```python
from build123d import *

# Parameters (mm, degrees)
SKETCH1_W                   = 231.775
SKETCH1_H                   = 298.45
BOSS_EXTRUDE1_DEPTH         = 3.175
F_1_4_0_25_DIAMETER_HOLE1_D = 6.35
FILLET1_R                   = 3.175
SKETCH4_W                   = 12.7
SKETCH4_H                   = 19.05
CUT_EXTRUDE1_DEPTH          = 4.175
FILLET2_R                   = 1.905


with BuildPart() as part:
    # Sketch1 → Boss-Extrude1 (new body)
    with BuildSketch(Plane(origin=(0, 0, 0), x_dir=(1, 0, 0), z_dir=(0, 1, 0))):
        Rectangle(SKETCH1_W, SKETCH1_H)
    extrude(amount=BOSS_EXTRUDE1_DEPTH)

    # 1/4 (0.25) Diameter Hole1 (through all)
    with Locations(Plane(origin=(0, 3.175, 0), x_dir=(1, 0, 0), z_dir=(0, 1, 0))):
        with Locations((61.9125, 0)):
            Hole(F_1_4_0_25_DIAMETER_HOLE1_D / 2)

    # Fillet1
    fillet1_edges = [part.edges().sort_by_distance(p)[0] for p in [
        (115.8875, 1.5875, 149.225),
        (-115.8875, 1.5875, 149.225),
        (-115.8875, 1.5875, -149.225),
        (115.8875, 1.5875, -149.225),
    ]]
    fillet(fillet1_edges, radius=FILLET1_R)

    # Sketch4 → Cut-Extrude1 (cut, through all)
    with BuildSketch(Plane(origin=(0, 3.175, 0), x_dir=(1, 0, 0), z_dir=(0, 1, 0))):
        with Locations((61.9125, -114.3)):
            Rectangle(SKETCH4_W, SKETCH4_H)
        with Locations((61.9125, 114.3)):
            Rectangle(SKETCH4_W, SKETCH4_H)
    extrude(amount=-CUT_EXTRUDE1_DEPTH, mode=Mode.SUBTRACT)

    # Fillet2
    fillet2_edges = [part.edges().sort_by_distance(p)[0] for p in [
        (55.5625, 1.5875, 123.825),
        (55.5625, 1.5875, 104.775),
        (68.2625, 1.5875, 104.775),
        (68.2625, 1.5875, 123.825),
        (55.5625, 1.5875, -104.775),
        (55.5625, 1.5875, -123.825),
        (68.2625, 1.5875, -123.825),
        (68.2625, 1.5875, -104.775),
    ]]
    fillet(fillet2_edges, radius=FILLET2_R)


solid = part.part
```
CAD build for the part. Positions are in the model's coordinates, mm. Give positions to 0.01 mm unless a question says otherwise; leave off trailing zeros. Order: outer loops, then holes, each group sorted by start corner. A loop starts at its lowest first (then second) coordinate and runs counter-clockwise, first axis right, second up. Notation, with made-up numbers: M 55,-17.75 L 97,-17.75 A7 cw 97,-11.75 Z; hole C 31,15 d10. An arc over 180 degrees is marked long. Put each result on its own line as item: value. Start each with the question number.
(1) Saw through at A-A, the plane z = -117.5. Write the cut outline in (x, y) (1 decimal), then the cut area to 3 significant figures.
(2) Drill centre lines: line 1 along X through (y, z) = (0.2, -115); line 2 along X through (y, z) = (2.75, 2). Where is each one in solid material? Low to high.
(3) Saw through at B-B, the plane z = 0. Write the cut outline in (x, y) (1 decimal), then the cut area to 3 significant figures.
(4) Mould opens along X. For faces 1 (the flat face through (-2, 3.175, -2)), 2 (the cylindrical face through (65.084, 1.565, -0.14)) say: +X half, -X half, draft (parallel to the pull), parting line (faces both ways), or undercut.
Check result:
1. outline: M -115.9,0 L 55.6,0 L 55.6,3.2 L -115.9,3.2 Z; M 68.3,0 L 115.9,0 L 115.9,3.2 L 68.3,3.2 Z
1. area: 696 mm2
2. line 1: x = -115.89 to 55.56, 68.26 to 115.89
2. line 2: x = -115.89 to 59.45, 64.38 to 115.89
3. outline: M -115.9,0 L 58.7,0 L 58.7,3.2 L -115.9,3.2 Z; M 65.1,0 L 115.9,0 L 115.9,3.2 L 65.1,3.2 Z
3. area: 716 mm2
4. face 1: draft
4. face 2: undercut
